The listing builds one solid part. Answer for the finished solid, in the listing's coordinates (mm). Round coordinates to 2 decimals unless told otherwise and drop trailing zeros. Write each loop counter-clockwise with the first axis right and the second up, starting at its lowest first coordinate (ties: lowest second). Pieces come first, ordered by that corner, then holes. Notation, with made-up numbers: M -14,-4.5 L -6,-4.5 A10 ccw -6,8.5 Z; hole C -32.5,13 d8. An arc over 180 degrees is marked long. One line per item, written item: value. Start each with the question number.
(1) Section B-B (x = 39.96) is taken. Determine the outline of the cut face in (y, z), plus the area to 3 significant figures.
(2) Given P1, Ø3, axis at x = -41, y = 1, coming from the +Z side, flat-ended and moving along its own axis, determine where the tip first touches the part or whether it passes through.
(3) Consider probe 1 along X at (y, z) = (-0.04, 7.9); probe 2 along X at (y, z) = (-0.04, 4.5); probe 3 along Y at (x, z) = (39.96, 4.5). Determine where each line is inside the solid, lowest interval first.
(4) Section C-C (z = 7.75) is taken. Determine the outline of the cut face in (x, y), plus the area to 3 significant figures.
(5) Section A-A (y = -0.04) is taken. Determine the outline of the cut face in (x, z), plus the area to 3 significant figures.
(6) Section D-D (z = 3) is taken. Determine the outline of the cut face in (x, y), plus the area to 3 significant figures.
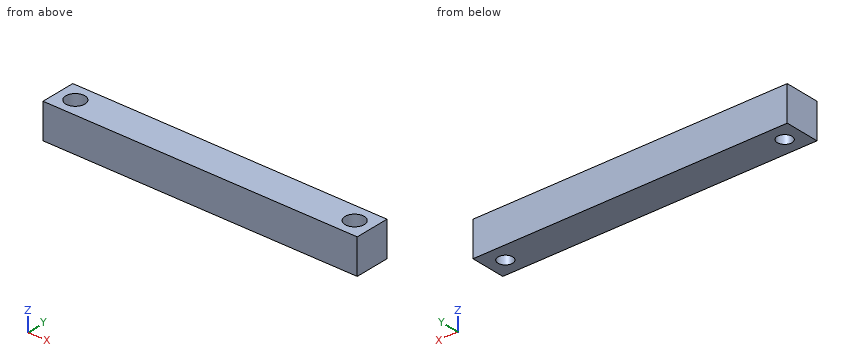
Autodesk Fusion 360 part; units mm, degrees
sketch "Sketch1" plane through (0, 0, 0) normal (0, 0, 1) x (1, 0, 0)
  line L0 (-45, -5) -> (45, -5)
  line L1 (45, -5) -> (45, 5)
  line L2 (45, 5) -> (-45, 5)
  line L3 (-45, 5) -> (-45, -5)
  line L4 (-45, -5) -> (45, 5) construction
  line L5 (45, -5) -> (-45, 5) construction
  dimension "d1" = 90
  dimension "d2" = 10
extrude "Extrude1" add sketch "Sketch1" along normal blind 10
sketch "Sketch2" plane through (0, 0, 10) normal (0, 0, 1) x (-1, 0, 0)
  line L0 (45, -5) -> (45, 5)
  line L1 (45, 5) -> (-45, 5)
  line L2 (-45, 5) -> (-45, -5)
  line L3 (-45, -5) -> (45, -5)
  circle A0 centre (-40, 0) radius 2.75
  circle A1 centre (-40, 0) radius 2.1
  dimension "d5" = 5.5
  dimension "d6" = 4.2
  dimension "d7" = 5
  dimension "d8" = 5
extrude "Extrude2" cut sketch "Sketch2" against normal blind 10 contours A1
extrude "Extrude3" cut sketch "Sketch2" against normal blind 4 contours A0
mirror "Mirror1" about plane through (0, 0, 0) normal (1, 0, 0) of "Extrude2", "Extrude3"
scale "Scale1" factor 1.008 about (45, 5, 0) bodies 1
Recorded:
1. outline: M -5.08,0 L -2.16,0 L -2.16,6.05 L -2.81,6.05 L -2.81,10.08 L -5.08,10.08 Z; M 2.08,0 L 5,0 L 5,10.08 L 2.73,10.08 L 2.73,6.05 L 2.08,6.05 Z
1. area: 53.6 mm2
2. P1: stops at z = 6.05
3. probe 1: x = -45.72 to -43.45, -37.91 to 37.19, 42.73 to 45
3. probe 2: x = -45.72 to -42.8, -38.56 to 37.84, 42.08 to 45
3. probe 3: y = -5.08 to -2.16, 2.08 to 5
4. outline: M -45.72,-5.08 L 45,-5.08 L 45,5 L -45.72,5 Z; hole C -40.68,-0.04 d5.54; hole C 39.96,-0.04 d5.54
4. area: 866 mm2
5. outline: M -45.72,0 L -42.8,0 L -42.8,6.05 L -43.45,6.05 L -43.45,10.08 L -45.72,10.08 Z; M -38.56,0 L 37.84,0 L 37.84,6.05 L 37.19,6.05 L 37.19,10.08 L -37.91,10.08 L -37.91,6.05 L -38.56,6.05 Z; M 42.08,0 L 45,0 L 45,10.08 L 42.73,10.08 L 42.73,6.05 L 42.08,6.05 Z
5. area: 819 mm2
6. outline: M -45.72,-5.08 L 45,-5.08 L 45,5 L -45.72,5 Z; hole C -40.68,-0.04 d4.23; hole C 39.96,-0.04 d4.23
6. area: 886 mm2
